from build123d import *

# Parameters (mm, degrees)
BOSS_EXTRUDE1_DEPTH = 6.35
SKETCH2_R           = 3.175
CUT_EXTRUDE1_DEPTH  = 76.2
FILLET1_R           = 58.42


with BuildPart() as part:
    # Sketch1 → Boss-Extrude1 (new body)
    with BuildSketch(Plane.XY):
        with BuildLine():
            add(Edge.make_bspline(
                [(0, 0), (38.404098046, -21.59977719), (31.400899659, -48.21557496)],
                knots=[0, 0, 0, 0.881342447, 0.881342447, 0.881342447], degree=2))
            add(Edge.make_bspline(
                [(0, 0), (-45.575290821, 25.610850897), (-36.060387995, 61.383694171)],
                knots=[0, 0, 0, 1, 1, 1], degree=2))
            add(Edge.make_bspline(
                [(-36.060387995, 61.383694171), (-62.615286542, 34.594392179), (-74.116408577, -18.870814993), (-51.051785251, -51.254371701)],
                knots=[0, 0, 0, 0, 1, 1, 1, 1], degree=3))
            add(Edge.make_bspline(
                [(-51.051785251, -51.254371701), (12.058894693, -90.706625614), (28.692128455, -55.473211038)],
                knots=[0, 0, 0, 0.914335656, 0.914335656, 0.914335656], degree=2))
            add(Edge.make_bspline(
                [(28.692128455, -55.473211038), (30.250500418, -52.172183336), (31.400899659, -48.21557496)],
                knots=[0.914335656, 0.914335656, 0.914335656, 1, 1, 1], degree=2))
        make_face()
    extrude(amount=BOSS_EXTRUDE1_DEPTH)

    # Sketch2 → Cut-Extrude1 (cut)
    with BuildSketch(Plane.XY.offset(6.35)):
        with Locations((-3.152469771, -38.871385351)):
            Circle(SKETCH2_R)
    extrude(amount=-CUT_EXTRUDE1_DEPTH, mode=Mode.SUBTRACT)

    # Fillet1
    fillet1_edges = [part.edges().sort_by_distance(p)[0] for p in [
        (-51.051785251, -51.254371701, 3.175),
    ]]
    fillet(fillet1_edges, radius=FILLET1_R)


solid = part.part
Can you work these out from the model? Positions are in its coordinate system, mm. Round coordinates to 2 decimals unless told otherwise and drop trailing zeros. Answer in a Markdown table with one row per item. Add a question column.
Q1. I need wall thicknesses on L1, parallel to Y at x = -49, z = 1; L2, parallel to X at y = -63, z = 4; L3, parallel to Y at x = 5.5, z = 2.75. Which ranges of each line are inside material? Lowest first, please.
Q2. We'd pull the mould along X, two halves only. Please class faces 1 (the flat face through (-24, -27, 0)), 2 (the cylindrical face through (-3.566, -35.723, 3.219)): pulls with the +X half, pulls with the -X half, needs draft (parallel to the pull), parting line crosses it, or undercut.
Q3. For pin 1 Ø3 at (x, z) = (-20, 4) entering from +Y; pin 2 Ø8.5 at (x, y) = (-3.15, -38.87) entering from -Z, each with a flat end and sliding along its axis, tell me the tip position at first contact or that it passes through.
A:
| question | item | result |
|---|---|---|
| 1 | L1 | -48.59 to 44.3 |
| 1 | L2 | -29.92 to 23.91 |
| 1 | L3 | -71.99 to -3.26 |
| 2 | face 1 | needs draft |
| 2 | face 2 | undercut |
| 3 | pin 1 | y = 15.42 |
| 3 | pin 2 | z = 0 |
